The listing builds one solid part. Answer for the finished solid, in the listing's coordinates (mm). Face numbers are marked on the shaded views. A direction names the side the tool comes from. Give positions to 0.01 mm unless a question says otherwise; leave off trailing zeros. Loops run counter-clockwise (first coordinate to the right, second up) from the corner with the lowest first, then second, coordinate; pieces in that order, holes last. Notation, with made-up numbers: (28, 80) - (65, 80) arc R20 ccw to (65, 118) - close; hole circle Ø10 at (-39, -36). An arc over 180 degrees is marked (long way). One line per item, written item: value. Start each with the question number.
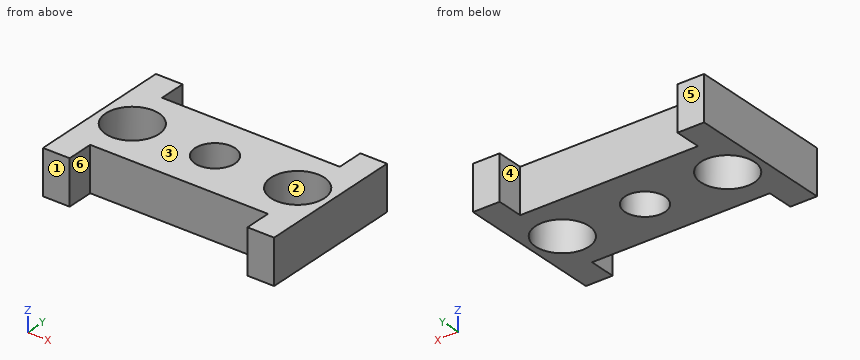
from build123d import *

# Parameters (mm, degrees)
SKETCH1_R           = 3
SKETCH1_R_2         = 2.25
BOSS_EXTRUDE1_DEPTH = 5


with BuildPart() as part:
    # Sketch1 → Boss-Extrude1 (new body)
    with BuildSketch(Plane.XY):
        Polygon((-13, 8.25), (-13, -8.25), (-10, -8.25), (-10, -5.25), (10, -5.25), (10, -8.25), (13, -8.25), (13, 8.25), (10, 8.25), (10, 5.25), (-10, 5.25), (-10, 8.25), align=None)
        with Locations((-9.3, 0)):
            Circle(SKETCH1_R, mode=Mode.SUBTRACT)
        Circle(SKETCH1_R_2, mode=Mode.SUBTRACT)
        with Locations((9.3, 0)):
            Circle(SKETCH1_R, mode=Mode.SUBTRACT)
    extrude(amount=BOSS_EXTRUDE1_DEPTH)


solid = part.part
1. A cutting plane is placed at A-A (x = 7.5). Determine the outline of the cut face in (y, z).
2. Flat-ended cylindrical pins translate along their axes: pin 1 (1.5 mm diameter, centred on x = -3.5, z = 1.5, fed in from -Y); pin 2 (2.5 mm diameter, centred on x = 1.5, z = 3.5, fed in from +Y); pin 3 (9.5 mm diameter, centred on x = -9.3, y = 0, fed in from +Z). Find the tip coordinate at first contact, or state that the pin passes through.
3. Determine the mould class of the marked faces 1, 2 and 3 for opening direction Y: released by +Y, released by -Y, zero draft, split by the parting line, or undercut.
4. For the marked faces 4, 5 and 6, determine the directions among +Z, -Z, +X, -X, +Y, -Y from which every point of the face is accessible in a straight line to the end or side of a thin tool.
5. A cutting plane is placed at B-B (y = 0). Determine the outline of the cut face in (x, z), plus the area to 3 significant figures.
6. Find the intervals of material crossed by L1, parallel to X at y = 5.75, z = 2.8; L2, parallel to Y at x = 0, z = 2.2; L3, parallel to X at y = 1, z = 1.2, in increasing order. Write a range as [from, to].
7. A cutting plane is placed at C-C (y = 6.5). Determine the outline of the cut face in (x, z), plus the area to 3 significant figures.
8. A cutting plane is placed at D-D (z = 2.9). Determine the outline of the cut face in (x, y), plus the area to 3 significant figures.
Results below:
1. outline: (-5.25, 0) - (-2.4, 0) - (-2.4, 5) - (-5.25, 5) - close; (2.4, 0) - (5.25, 0) - (5.25, 5) - (2.4, 5) - close
2. pin 1: stops at y = -5.25
2. pin 2: stops at y = 5.25
2. pin 3: stops at z = 5
3. face 1: released by -Y
3. face 2: undercut
3. face 3: zero draft
4. face 4: +Z, -Z, +Y
4. face 5: +Z, -Z, +X, -X, +Y
4. face 6: +Z, -Z, -Y
5. outline: (-13, 0) - (-12.3, 0) - (-12.3, 5) - (-13, 5) - close; (-6.3, 0) - (-2.25, 0) - (-2.25, 5) - (-6.3, 5) - close; (2.25, 0) - (6.3, 0) - (6.3, 5) - (2.25, 5) - close; (12.3, 0) - (13, 0) - (13, 5) - (12.3, 5) - close
5. area: 47.5 mm^2
6. L1: x = [-13, -10], [10, 13]
6. L2: y = [-5.25, -2.25], [2.25, 5.25]
6. L3: x = [-13, -12.13], [-6.47, -2.02], [2.02, 6.47], [12.13, 13]
7. outline: (-13, 0) - (-10, 0) - (-10, 5) - (-13, 5) - close; (10, 0) - (13, 0) - (13, 5) - (10, 5) - close
7. area: 30.0 mm^2
8. outline: (-13, -8.25) - (-10, -8.25) - (-10, -5.25) - (10, -5.25) - (10, -8.25) - (13, -8.25) - (13, 8.25) - (10, 8.25) - (10, 5.25) - (-10, 5.25) - (-10, 8.25) - (-13, 8.25) - close; hole circle Ø6 at (-9.3, 0); hole circle Ø4.5 at (0, 0); hole circle Ø6 at (9.3, 0)
8. area: 237 mm^2
